Design review of the part built by this model. Coordinates are the model's own, in mm. A direction names the side the tool comes from. Coordinates: 2 decimals unless noted, no trailing zeros. Loops run counter-clockwise (first coordinate to the right, second up) from the corner with the lowest first, then second, coordinate; pieces in that order, holes last. Notation, with made-up numbers: M 15,72 L 50,72 A28 ccw 50,106 Z; hole C 84.25,19.5 d3. An arc over 180 degrees is marked long. Answer as a JSON object with one key per item and string values. Group by question number.
1. Consider section B-B (z = 95.5). State the section outline as (x, y) points, then the cut area to 3 significant figures.
2. To check wall thickness, follow probe 1 along Z at (x, y) = (-262.5, -7.75); probe 2 along Z at (x, y) = (236, -8.5); probe 3 along X at (y, z) = (-6, -43). State the ranges of each line that lie inside material, in increasing order.
3. Consider section D-D (z = 212). State the section outline as (x, y) points.
4. Machinability: for faces 4 (the flat face through (168, 0, -311)), 5 (the cylindrical face through (-339.87, -4.93, -122.3)), which of the approach directions +Z, -Z, +X, -X, +Y, -Y give a long, thin tool a straight path to every point of the face, cutting with its end or side? Answer none if there is none.
5. Insertion check: pin 1 (1 mm diameter, centred on y = -5, z = 342.5, fed in from +X); pin 2 (2 mm diameter, centred on x = -167, y = -2, fed in from +Z); pin 3 (6 mm diameter, centred on y = -7, z = 294.5, fed in from +X). Each pin has a flat end and moves straight along its axis. Give the tip position at first contact, or say it passes through.
6. Draft analysis for pull direction Z (two halves, no side actions). For faces 1 (the flat face through (168, -10, -311)), 2 (the cylindrical face through (310, -4.9, 97.6)), 3 (the cylindrical face through (368.461, -4.93, 337.272)), state which applies: +Z half, -Z half, draft (parallel to the pull), parting line (faces both ways), or undercut.
7. Consider section C-C (x = 341). State the section outline as (y, z) points, then the cut area to 3 significant figures.
8. Consider section A-A (y = -6.5). State the section outline as (x, z) points.
from build123d import *

# Parameters (mm, degrees)
F0_R     = 325
F1_DEPTH = 10


# Not quite as in the source:
# - a feature names something its author has since deleted; it is built from what else it names


with BuildPart() as f1:
    # F0 (on Front) → F1 (new body)
    with BuildSketch(Plane.XZ):
        with BuildLine():
            ThreePointArc((0, -618.6190456596), (397.429722157, -420.8611796621), (538.6190456596, 0))
            ThreePointArc((538.6190456596, 0), (364.2926371672, 340.8611796621), (0, 458.6190456596))
            ThreePointArc((0, 458.6190456596), (-284.2926371672, 307.7240946723), (-378.6190456596, 0))
            ThreePointArc((-378.6190456596, 0), (-338.9932719851, -123.9081492515), (-255.845498181, -223.9575325662))
            Line((-255.845498181, -223.9575325662), (-248.8807463186, -229.5026751274))
            ThreePointArc((-248.8807463186, -229.5026751274), (-232.823383589, -285.1142187928), (-280.0241173048, -318.6190456596))
            Line((-280.0241173048, -318.6190456596), (-400, -318.6190456596))
            Line((-400, -318.6190456596), (-400, -618.6190456596))
            Line((-400, -618.6190456596), (0, -618.6190456596))
        make_face()
        Circle(F0_R, mode=Mode.SUBTRACT)
    extrude(amount=F1_DEPTH)


solid = f1.part
Findings below:
{
 "1": {"outline": "M -376.85,-10 L -310.65,-10 L -310.65,0 L -376.85,0 Z; M 310.65,-10 L 521.52,-10 L 521.52,0 L 310.65,0 Z", "area": "2,770 mm^2"},
 "2": {"probe 1": "z = -618.62 to -315.45, -218.37 to -191.62, 191.62 to 332.12", "probe 2": "z = -550.12 to -223.45, 223.45 to 420.22", "probe 3": "x = -370.72 to -322.14, 322.14 to 539.99"},
 "3": {"outline": "M -343.74,-10 L -246.34,-10 L -246.34,0 L -343.74,0 Z; M 246.34,-10 L 472.11,-10 L 472.11,0 L 246.34,0 Z"},
 "4": {"face 4": "+Z, -Z, +X, -X, +Y", "face 5": "-X, +Y, -Y"},
 "5": {"pin 1": "stops at x = 362.95", "pin 2": "stops at z = 406.61", "pin 3": "stops at x = 414.6"},
 "6": {"face 1": "draft", "face 2": "undercut", "face 3": "+Z half"},
 "7": {"outline": "M -10,-477.31 L 0,-477.31 L 0,359.52 L -10,359.52 Z", "area": "8,370 mm^2"},
 "8": {"outline": "M -400,-618.62 L 0,-618.62 A580 ccw 538.62,0 A500.22 ccw 0,458.62 A420.53 ccw -378.62,0 A340.97 ccw -255.85,-223.96 L -248.88,-229.5 A50 cw -280.02,-318.62 L -400,-318.62 Z; hole C 0,0 d650"}
}
